Check sheet for the modelled part. Datum: model origin and axes. Units: mm. Face numbers are marked on the shaded views. A direction names the side the tool comes from. Coordinates: 2 decimals unless noted, no trailing zeros. Write each loop counter-clockwise with the first axis right and the second up, starting at its lowest first coordinate (ties: lowest second). Pieces come first, ordered by that corner, then holes. Notation, with made-up numbers: M -13,24 L 25,24 A7 ccw 25,28 Z; hole C 5,-14.5 d10. An arc over 180 degrees is marked long. Answer as CSV lines item,"result". Start each with the question number.
1) Access from +Z, -Z, +X, -X, +Y, -Y to the whole of each face (thin tool, end or side, straight path). Record for the marked faces 4 and 5.
2) Section check C-C (y = 0). Record the cut outline in (x, z), and give its area (3 significant figures).
3) Material ranges on L1, parallel to Z at x = 1.5, y = -2.25; L2, parallel to X at y = 1.25, z = 19.75; L3, parallel to X at y = 1.5, z = 13, recorded low to high. Write a range as [from, to].
4) Section check D-D (z = 17.25). Record the cut outline in (x, y), and give its area (3 significant figures).
5) Go/stop test with flat-tipped pins: pin 1 Ø3.5 at (x, y) = (0.5, -0.5) entering from +Z; pin 2 Ø3 at (x, y) = (-1.5, 0) entering from -Z; pin 3 Ø5 at (y, z) = (-3, 4.5) entering from -X; pin 4 Ø1.5 at (x, y) = (0, 1) entering from +Z. Record where each tip stops, or that it passes through.
6) Section check B-B (x = 0). Record the cut outline in (y, z), and give its area (3 significant figures).
7) Draft check along X on the marked faces 1, 2 and 3. Enter one of: +X half, -X half, draft (parallel to the pull), parting line (faces both ways), or undercut.
8) Section check A-A (z = 7). Record the cut outline in (x, y).
Solid Edge part; units mm, degrees
sketch "Sketch1" plane through (0, 0, 0) normal (0, -1, 0) x (1, 0, 0)
  line L0 (2.5, 16) -> (2.5, 0)
  line L1 (2.5, 0) -> (0, 0)
  line L2 (0, 0) -> (0, 21)
  line L3 (0, 21) -> (4.25, 21)
  line L4 (4.25, 21) -> (4.25, 16)
  line L5 (4.25, 16) -> (2.5, 16)
revolve "RevolvedProtrusion1" add sketch "Sketch1" angle 360 about axis through (0, 0, 0) along (0, 0, 1)
sketch "Sketch2" plane through (0, 0, 21) normal (0, 0, 1) x (1, 0, 0)
  line L0 (0.9623, -2.0994) -> (2.2992, -0.2164)
  line L1 (2.2992, -0.2164) -> (1.337, 1.883)
  line L2 (1.337, 1.883) -> (-0.9623, 2.0994)
  line L3 (-0.9623, 2.0994) -> (-2.2992, 0.2164)
  line L4 (-2.2992, 0.2164) -> (-1.337, -1.883)
  line L5 (-1.337, -1.883) -> (0.9623, -2.0994)
extrude "Cutout1" cut sketch "Sketch2" against normal blind 2.5
cosmetic_thread "Thread1"
chamfer "Chamfer1" distance 0.5 angle 45 9 edges at (-4.25, 0, 16) (-4.25, 0, 21) (-2.5, 0, 0) (1.8181, 0.8333, 21) (0.1874, 1.9912, 21) (-1.6307, 1.1579, 21) (-1.8181, -0.8333, 21) (-0.1874, -1.9912, 21) (1.6307, -1.1579, 21)
properties material "Stainless steel"
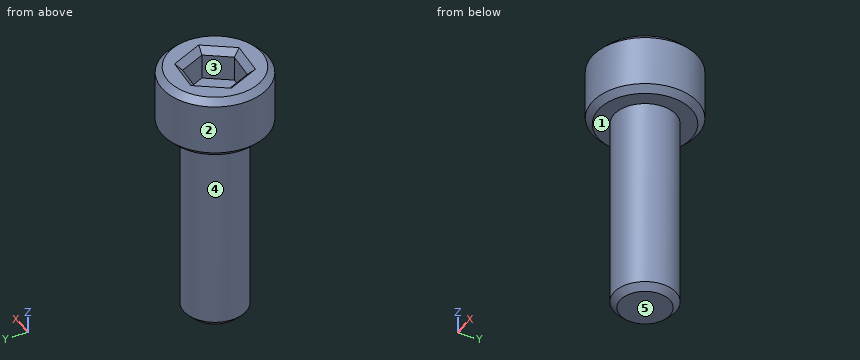
Results found:
1,face 4,"-Z"
1,face 5,"-Z, +X, -X, +Y, -Y"
2,outline,"M -4.25,16.5 L -3.75,16 L -2.5,16 L -2.5,0.5 L -2,0 L 2,0 L 2.5,0.5 L 2.5,16 L 3.75,16 L 4.25,16.5 L 4.25,20.5 L 3.75,21 L 2.75,21 L 2.2,20.5 L 2.2,18.5 L -2.2,18.5 L -2.2,20.5 L -2.75,21 L -3.75,21 L -4.25,20.5 Z"
2,area,"110 mm2"
3,L1,"z = [16, 21]"
3,L2,"x = [-4.06, -1.57], [1.63, 4.06]"
3,L3,"x = [-2, 2]"
4,outline,"C 0,0 d8.5"
4,area,"56.7 mm2"
5,pin 1,"stops at z = 20.95"
5,pin 2,"stops at z = 0"
5,pin 3,"stops at x = -2.45"
5,pin 4,"stops at z = 18.5"
6,outline,"M -4.25,16.5 L -3.75,16 L -2.5,16 L -2.5,0.5 L -2,0 L 2,0 L 2.5,0.5 L 2.5,16 L 3.75,16 L 4.25,16.5 L 4.25,20.5 L 3.75,21 L 2.51,21 L 2.01,20.5 L 2.01,18.5 L -2.01,18.5 L -2.01,20.5 L -2.51,21 L -3.75,21 L -4.25,20.5 Z"
6,area,"111 mm2"
7,face 1,"draft"
7,face 2,"parting line"
7,face 3,"undercut"
8,outline,"C 0,0 d5"
